Read the model definition and answer for the solid it produces. Units are mm, in the model's axes. Coordinates: 2 decimals unless noted, no trailing zeros. Order: outer loops, then holes, each group sorted by start corner. A loop starts at its lowest first (then second) coordinate and runs counter-clockwise, first axis right, second up. Notation, with made-up numbers: (3, -27) -> (31, -27) arc R15 cw to (31, -3) -> close; hole circle Ø11 at (60.5, -25.5). An arc over 180 degrees is marked (long way). Answer in a Markdown table with one row per item.
from build123d import *

# Parameters (mm, degrees)
F0_W     = 60.96
F0_H     = 63.5
F0_R     = 6.35
F1_DEPTH = 2.54
F2_R     = 1.26999


# Not quite as in the source:
# - a fillet or chamfer is up to 0.001 mm smaller than in the source, because OpenCascade refuses the exact size


with BuildPart() as f1:
    # F0 (on Top) → F1 (new body)
    with BuildSketch(Plane.XY):
        Rectangle(F0_W, F0_H)
        Circle(F0_R, mode=Mode.SUBTRACT)
    extrude(amount=F1_DEPTH)

    # F2 (radius 1.27 in the source; OpenCascade refuses exactly that, so slightly less here)
    f2_edges = [f1.edges().sort_by_distance(p)[0] for p in [
        (-6.35, 0, 2.54),
        (-6.35, 0, 0),
    ]]
    fillet(f2_edges, radius=F2_R)


solid = f1.part
Q1. Given pin 1 (10 mm diameter, centred on x = 0, y = 0, fed in from +Z), flat-ended and moving along its own axis, determine where the tip first touches the part or whether it passes through.
Outcome:
| item | result |
|---|---|
| pin 1 | through |
Q2. The part is cut by section C-C (z = 0.5). Write down the section's boundary in (x, y), then the cut area to 3 significant figures.
Outcome:
| item | result |
|---|---|
| outline | (-30.48, -31.75) -> (30.48, -31.75) -> (30.48, 31.75) -> (-30.48, 31.75) -> close; hole circle Ø13.22 at (0, 0) |
| area | 3,730 mm² |
Q3. Consider line 1 (Y direction, x = 0, z = 1.3); line 2 (X direction, y = -0.5, z = 0.55); line 3 (Y direction, x = 4.5, z = 1.2). Determine where each line is inside the solid, lowest interval first.
Outcome:
| item | result |
|---|---|
| line 1 | -31.75 to -6.35, 6.35 to 31.75 |
| line 2 | -30.48 to -6.55, 6.55 to 30.48 |
| line 3 | -31.75 to -4.48, 4.48 to 31.75 |
